Source: CAD feature listing. Evaluate the final solid. Frame: model axes, mm. Coordinates: 2 decimals unless noted, no trailing zeros. Order: outer loops, then holes, each group sorted by start corner. A loop starts at its lowest first (then second) coordinate and runs counter-clockwise, first axis right, second up.
```python
from build123d import *

# Parameters (mm, degrees)
F1_DEPTH = 40
F2_SIZE  = 1


with BuildPart() as f1:
    # F0 (on Top) → F1 (new body)
    with BuildSketch(Plane.XY):
        Polygon((2.864027, -1.186319), (2.864027, 1.186319), (1.186319, 2.864027), (-1.186319, 2.864027), (-2.864027, 1.186319), (-2.864027, -1.186319), (-1.186319, -2.864027), (1.186319, -2.864027), align=None)
    extrude(amount=F1_DEPTH)

    # F2
    f2_edges = [f1.edges().sort_by_distance(p)[0] for p in [
        (2.025173, -2.025173, 40),
        (2.864027, 0, 40),
        (2.025173, 2.025173, 40),
        (0, 2.864027, 40),
        (-2.025173, 2.025173, 40),
        (-2.864027, 0, 40),
        (-2.025173, -2.025173, 40),
        (0, -2.864027, 40),
        (2.025173, -2.025173, 0),
        (2.864027, 0, 0),
        (2.025173, 2.025173, 0),
        (0, 2.864027, 0),
        (-2.025173, 2.025173, 0),
        (-2.864027, 0, 0),
        (-2.025173, -2.025173, 0),
        (0, -2.864027, 0),
    ]]
    chamfer(f2_edges, length=F2_SIZE)


solid = f1.part
```
1. Contact query for a flat-ended pin moving along its axis: P1, Ø1, axis at y = 2, z = 36, coming from the -X side. Output: stop coordinate, or through.
2. Section query A-A, the plane z = 16. Output: boundary loops of the cut face in (x, y), plus the area to 3 significant figures.
3. Material intervals for line 1 along Z through (x, y) = (-1.6, -1.15); line 2 along Y through (x, z) = (2.45, 4); line 3 along Y through (x, z) = (-1.3, 11.5), sorted ascending.
Answer key:
1. P1: stops at x = -2.55
2. outline: (-2.86, -1.19) - (-1.19, -2.86) - (1.19, -2.86) - (2.86, -1.19) - (2.86, 1.19) - (1.19, 2.86) - (-1.19, 2.86) - (-2.86, 1.19) - close
2. area: 27.2 mm2
3. line 1: z = 0.08 to 39.92
3. line 2: y = -1.6 to 1.6
3. line 3: y = -2.75 to 2.75
